Model file for the job. Use its own axes, mm. A direction names the side the tool comes from. Round coordinates to 2 decimals unless told otherwise and drop trailing zeros. Order: outer loops, then holes, each group sorted by start corner. A loop starts at its lowest first (then second) coordinate and runs counter-clockwise, first axis right, second up. Notation, with made-up numbers: (60, 28.5) - (89, 28.5) arc R20 ccw to (89, 47.5) - close; hole circle Ø5 at (36.25, -15.5). An arc over 180 degrees is marked (long way). Put each result on its own line as item: value. Start each with the question number.
Item 1: Saw through at C-C on x = 0. List the corners of the cut face in (y, z), plus the area to 3 significant figures.
Item 2: Saw through at B-B on z = 0.5. List the corners of the cut face in (x, y), plus the area to 3 significant figures.
Item 3: Saw through at A-A on x = -4. List the corners of the cut face in (y, z), plus the area to 3 significant figures.
Item 4: Mould opens along X. For faces 1 (the face through (0, 0, -6)), 2 (the face through (13.815, 2.507, 7.799)), 3 (the face through (15.43, 1.52, 11.9)) say: pulls with the +X half, pulls with the -X half, needs draft (parallel to the pull), parting line crosses it, or undercut.
Item 5: Pin check, flat tips, straight feed: pin 1 Ø1 at (x, z) = (9, 7) entering from +Y; pin 2 Ø1.8 at (x, z) = (10, 6.5) entering from +Y. Stop position of each tip, or through.
Item 6: Which spindle directions (+Z, -Z, +X, -X, +Y, -Y) get a long thin tool onto all of the face, cutting with end or side? Do faces 4 (the face through (11.799, 2.507, -2.685)), 5 (the face through (0, 1, 12.5)), 6 (the face through (7.5, 2, 0)). Say none if no direction does.
Item 7: Probe probe 1 along Z at (x, y) = (0, 0.9); probe 2 along Z at (x, y) = (3, 2.05); probe 3 along X at (y, z) = (0.9, 1). List the from-to ranges inside material, lowest first.
```python
from build123d import *

# Parameters (mm, degrees)
SKETCH1_W                                      = 32
SKETCH1_H                                      = 25
BOSS_EXTRUDE1_DEPTH                            = 3
CUT_EXTRUDE1_DEPTH                             = 1
CUT_EXTRUDE2_REACH                             = 4
SKETCH3_R                                      = 1
CUT_EXTRUDE3_REACH                             = 5
SKETCH4_R                                      = 1
FILLET1_R                                      = 2
CUT_EXTRUDE4_REACH                             = 5
CSK_FOR_M2_FLAT_HEAD_MACHINE_SCREW5_AT_2_COUNT = 2
CSK_FOR_M2_FLAT_HEAD_MACHINE_SCREW5_AT_2_PITCH = 22
CSK_FOR_M2_FLAT_HEAD_MACHINE_SCREW5_AT_3_COUNT = 2
CSK_FOR_M2_FLAT_HEAD_MACHINE_SCREW5_AT_3_PITCH = 13.03840481
CSK_FOR_M2_FLAT_HEAD_MACHINE_SCREW5_AT_4_COUNT = 2
CSK_FOR_M2_FLAT_HEAD_MACHINE_SCREW5_AT_4_PITCH = 24.69817807


with BuildPart() as part:
    # Sketch1 → Boss-Extrude1 (new body)
    with BuildSketch(Plane(origin=(0, 0, 0), x_dir=(1, 0, 0), z_dir=(0, 1, 0))):
        Rectangle(SKETCH1_W, SKETCH1_H)
    extrude(amount=BOSS_EXTRUDE1_DEPTH)

    # Sketch2 → Cut-Extrude1 (cut)
    with BuildSketch(Plane(origin=(0, 3, 0), x_dir=(1, 0, 0), z_dir=(0, 1, 0))):
        with BuildLine():
            Line((14.1, -5.9), (14.1, -7.1))
            ThreePointArc((14.1, -7.1), (13.807106781, -7.807106781), (13.1, -8.1))
            Line((13.1, -8.1), (6.9, -8.1))
            ThreePointArc((6.9, -8.1), (6.192893219, -7.807106781), (5.9, -7.1))
            Line((5.9, -7.1), (5.9, -5.9))
            ThreePointArc((5.9, -5.9), (6.192893219, -5.192893219), (6.9, -4.9))
            Line((6.9, -4.9), (13.1, -4.9))
            ThreePointArc((13.1, -4.9), (13.807106781, -5.192893219), (14.1, -5.9))
        make_face()
        with BuildLine():
            Line((-13.1, -4.9), (-6.9, -4.9))
            ThreePointArc((-6.9, -4.9), (-6.192893219, -5.192893219), (-5.9, -5.9))
            Line((-5.9, -5.9), (-5.9, -7.1))
            ThreePointArc((-5.9, -7.1), (-6.192893219, -7.807106781), (-6.9, -8.1))
            Line((-6.9, -8.1), (-13.1, -8.1))
            ThreePointArc((-13.1, -8.1), (-13.807106781, -7.807106781), (-14.1, -7.1))
            Line((-14.1, -7.1), (-14.1, -5.9))
            ThreePointArc((-14.1, -5.9), (-13.807106781, -5.192893219), (-13.1, -4.9))
        make_face()
        with BuildLine():
            Line((11.1, 10.6), (10.9, 10.6))
            ThreePointArc((10.9, 10.6), (10.192893219, 10.307106781), (9.9, 9.6))
            Line((9.9, 9.6), (9.9, 3.4))
            ThreePointArc((9.9, 3.4), (10.192893219, 2.692893219), (10.9, 2.4))
            Line((10.9, 2.4), (11.1, 2.4))
            ThreePointArc((11.1, 2.4), (11.807106781, 2.692893219), (12.1, 3.4))
            Line((12.1, 3.4), (12.1, 9.6))
            ThreePointArc((12.1, 9.6), (11.807106781, 10.307106781), (11.1, 10.6))
        make_face()
        with BuildLine():
            Line((-11.1, 10.6), (-10.9, 10.6))
            ThreePointArc((-10.9, 10.6), (-10.192893219, 10.307106781), (-9.9, 9.6))
            Line((-9.9, 9.6), (-9.9, 3.4))
            ThreePointArc((-9.9, 3.4), (-10.192893219, 2.692893219), (-10.9, 2.4))
            Line((-10.9, 2.4), (-11.1, 2.4))
            ThreePointArc((-11.1, 2.4), (-11.807106781, 2.692893219), (-12.1, 3.4))
            Line((-12.1, 3.4), (-12.1, 9.6))
            ThreePointArc((-12.1, 9.6), (-11.807106781, 10.307106781), (-11.1, 10.6))
        make_face()
    extrude(amount=-CUT_EXTRUDE1_DEPTH, mode=Mode.SUBTRACT)

    # Sketch3 → Cut-Extrude2 (cut, up to next)
    with BuildSketch(Plane(origin=(0, 2, 0), x_dir=(1, 0, 0), z_dir=(0, 1, 0)), mode=Mode.PRIVATE) as cut_extrude2_sk1:
        with Locations((-10, -6.5)):
            Circle(SKETCH3_R)
    cut_extrude2_tool1 = extrude(cut_extrude2_sk1.sketch, amount=-CUT_EXTRUDE2_REACH, mode=Mode.PRIVATE) & part.part
    add(cut_extrude2_tool1.solids().sort_by_distance((-10, 2, 6.5))[0], mode=Mode.SUBTRACT)
    # Sketch3 → Cut-Extrude2 (cut, up to next)
    with BuildSketch(Plane(origin=(0, 2, 0), x_dir=(1, 0, 0), z_dir=(0, 1, 0)), mode=Mode.PRIVATE) as cut_extrude2_sk2:
        with Locations((10, -6.5)):
            Circle(SKETCH3_R)
    cut_extrude2_tool2 = extrude(cut_extrude2_sk2.sketch, amount=-CUT_EXTRUDE2_REACH, mode=Mode.PRIVATE) & part.part
    add(cut_extrude2_tool2.solids().sort_by_distance((10, 2, 6.5))[0], mode=Mode.SUBTRACT)
    # Sketch3 → Cut-Extrude2 (cut, up to next)
    with BuildSketch(Plane(origin=(0, 2, 0), x_dir=(1, 0, 0), z_dir=(0, 1, 0)), mode=Mode.PRIVATE) as cut_extrude2_sk3:
        with Locations((-11, 6.5)):
            Circle(SKETCH3_R)
    cut_extrude2_tool3 = extrude(cut_extrude2_sk3.sketch, amount=-CUT_EXTRUDE2_REACH, mode=Mode.PRIVATE) & part.part
    add(cut_extrude2_tool3.solids().sort_by_distance((-11, 2, -6.5))[0], mode=Mode.SUBTRACT)
    # Sketch3 → Cut-Extrude2 (cut, up to next)
    with BuildSketch(Plane(origin=(0, 2, 0), x_dir=(1, 0, 0), z_dir=(0, 1, 0)), mode=Mode.PRIVATE) as cut_extrude2_sk4:
        with Locations((11, 6.5)):
            Circle(SKETCH3_R)
    cut_extrude2_tool4 = extrude(cut_extrude2_sk4.sketch, amount=-CUT_EXTRUDE2_REACH, mode=Mode.PRIVATE) & part.part
    add(cut_extrude2_tool4.solids().sort_by_distance((11, 2, -6.5))[0], mode=Mode.SUBTRACT)

    # Sketch4 → Cut-Extrude3 (cut, up to next)
    with BuildSketch(Plane(origin=(0, 3, 0), x_dir=(1, 0, 0), z_dir=(0, 1, 0)), mode=Mode.PRIVATE) as cut_extrude3_sk1:
        with Locations((0, 7.5)):
            Circle(SKETCH4_R)
    cut_extrude3_tool1 = extrude(cut_extrude3_sk1.sketch, amount=-CUT_EXTRUDE3_REACH, mode=Mode.PRIVATE) & part.part
    add(cut_extrude3_tool1.solids().sort_by_distance((0, 3, -7.5))[0], mode=Mode.SUBTRACT)

    # Sketch12 → CSK for M2 Flat Head Machine Screw4 (revolve, cut)
    with BuildSketch(Plane(origin=(0, 3, -7.5), x_dir=(0, 0, 1), z_dir=(1, 0, 0))):
        Polygon((0, 0), (0, 3), (1, 3), (1, 1.3), (2, 0.3), (2, 0), align=None)
    revolve(axis=Axis((0, 9.35, -7.5), (0, -1, 0)), mode=Mode.SUBTRACT)

    # Fillet1
    fillet1_edges = [part.edges().sort_by_distance(p)[0] for p in [
        (-16, 1.5, -12.5),
        (16, 1.5, -12.5),
        (16, 1.5, 12.5),
        (-16, 1.5, 12.5),
    ]]
    fillet(fillet1_edges, radius=FILLET1_R)

    # Sketch13 → Cut-Extrude4 (cut, up to next)
    with BuildSketch(Plane(origin=(0, 3, 0), x_dir=(1, 0, 0), z_dir=(0, 1, 0)), mode=Mode.PRIVATE) as cut_extrude4_sk1:
        with BuildLine():
            Line((6.5, 4), (-6.5, 4))
            ThreePointArc((-6.5, 4), (-7.207106781, 3.707106781), (-7.5, 3))
            Line((-7.5, 3), (-7.5, -3))
            ThreePointArc((-7.5, -3), (-7.207106781, -3.707106781), (-6.5, -4))
            Line((-6.5, -4), (6.5, -4))
            ThreePointArc((6.5, -4), (7.207106781, -3.707106781), (7.5, -3))
            Line((7.5, -3), (7.5, 3))
            ThreePointArc((7.5, 3), (7.207106781, 3.707106781), (6.5, 4))
        make_face()
    cut_extrude4_tool1 = extrude(cut_extrude4_sk1.sketch, amount=-CUT_EXTRUDE4_REACH, mode=Mode.PRIVATE) & part.part
    add(cut_extrude4_tool1.solids().sort_by_distance((0, 3, 0))[0], mode=Mode.SUBTRACT)

    # Sketch15 → CSK for M2 Flat Head Machine Screw5 (revolve, cut)
    with BuildSketch(Plane(origin=(11, 0, -6.5), x_dir=(0, 0, -1), z_dir=(1, 0, 0))):
        Polygon((0, 0), (0, 3), (1, 3), (1, 1.3), (2, 0.3), (2, 0), align=None)
    csk_for_m2_flat_head_machine_screw5 = revolve(axis=Axis((11, -6.35, -6.5), (0, 1, 0)), mode=Mode.SUBTRACT)

    # CSK for M2 Flat Head Machine Screw5 at 2: CSK for M2 Flat Head Machine Screw5 ×2
    with Locations(*[(-i * CSK_FOR_M2_FLAT_HEAD_MACHINE_SCREW5_AT_2_PITCH, 0, 0) for i in range(1, CSK_FOR_M2_FLAT_HEAD_MACHINE_SCREW5_AT_2_COUNT)]):
        add(csk_for_m2_flat_head_machine_screw5, mode=Mode.SUBTRACT)

    # CSK for M2 Flat Head Machine Screw5 at 3: CSK for M2 Flat Head Machine Screw5 ×2
    with Locations(*[Vector(-0.076696499, 0, 0.997054486) * (i * CSK_FOR_M2_FLAT_HEAD_MACHINE_SCREW5_AT_3_PITCH) for i in range(1, CSK_FOR_M2_FLAT_HEAD_MACHINE_SCREW5_AT_3_COUNT)]):
        add(csk_for_m2_flat_head_machine_screw5, mode=Mode.SUBTRACT)

    # CSK for M2 Flat Head Machine Screw5 at 4: CSK for M2 Flat Head Machine Screw5 ×2
    with Locations(*[Vector(-0.850265147, 0, 0.526354615) * (i * CSK_FOR_M2_FLAT_HEAD_MACHINE_SCREW5_AT_4_PITCH) for i in range(1, CSK_FOR_M2_FLAT_HEAD_MACHINE_SCREW5_AT_4_COUNT)]):
        add(csk_for_m2_flat_head_machine_screw5, mode=Mode.SUBTRACT)


solid = part.part
```
Results found:
1. outline: (0, -12.5) - (3, -12.5) - (3, -9.5) - (2.7, -9.5) - (1.7, -8.5) - (0, -8.5) - close; (0, -6.5) - (1.7, -6.5) - (2.7, -5.5) - (3, -5.5) - (3, -4) - (0, -4) - close; (0, 4) - (3, 4) - (3, 12.5) - (0, 12.5) - close
1. area: 43.4 mm²
2. outline: (-16, 0) - (-7.5, 0) - (-7.5, 3) - (-16, 3) - close; (7.5, 0) - (16, 0) - (16, 3) - (7.5, 3) - close
2. area: 51.0 mm²
3. outline: (0, -12.5) - (3, -12.5) - (3, -4) - (0, -4) - close; (0, 4) - (3, 4) - (3, 12.5) - (0, 12.5) - close
3. area: 51.0 mm²
4. face 1: needs draft
4. face 2: undercut
4. face 3: pulls with the +X half
5. pin 1: stops at y = 2
5. pin 2: passes through
6. face 4: +Y
6. face 5: +Z, +X, -X, +Y, -Y
6. face 6: +Y, -Y
7. probe 1: z = -12.5 to -8.5, -6.5 to -4, 4 to 12.5
7. probe 2: z = -12.5 to -4, 4 to 12.5
7. probe 3: x = -16 to -7.5, 7.5 to 16
